Geometry: see drawing. Coordinates: mm, zero at the bounding-box minimum. Coordinates: 2 decimals unless noted, no trailing zeros. Loops run counter-clockwise (first coordinate to the right, second up) from the corner with the lowest first, then second, coordinate; pieces in that order, holes last. Notation, with made-up numbers: (-25, 11) -> (12, 11) arc R24 cw to (12, 29) -> close; hole circle Ø3 at (83.25, 8.25). An arc over 180 degrees is marked (long way). Put each result on its own line as item: value. Start each with the question number.
1) Contact query for flat-ended pins moving along their axis: P1, Ø4, axis at x = 14.5, z = 20, coming from the +Y side; P2, Ø3, axis at x = 12, z = 27, coming from the +Y side; P3, Ø3, axis at y = 4, z = 19.5, coming from the -X side. Output: stop coordinate, or through.
2) Cut plane A-A (y = 10). Return the cut outline in (x, z).
3) Material intervals for L1, parallel to Y at x = 10, z = 23.25; L2, parallel to Y at x = 17, z = 28.5; L3, parallel to X at y = 9, z = 26.5, sorted ascending.
4) Pull-direction query (X, two-part tool) for the marked faces 1 and 2; classes: pulls with the +X half, pulls with the -X half, needs draft (parallel to the pull), parting line crosses it, or undercut.
5) Cut plane C-C (z = 14.5). Return the cut outline in (x, y).
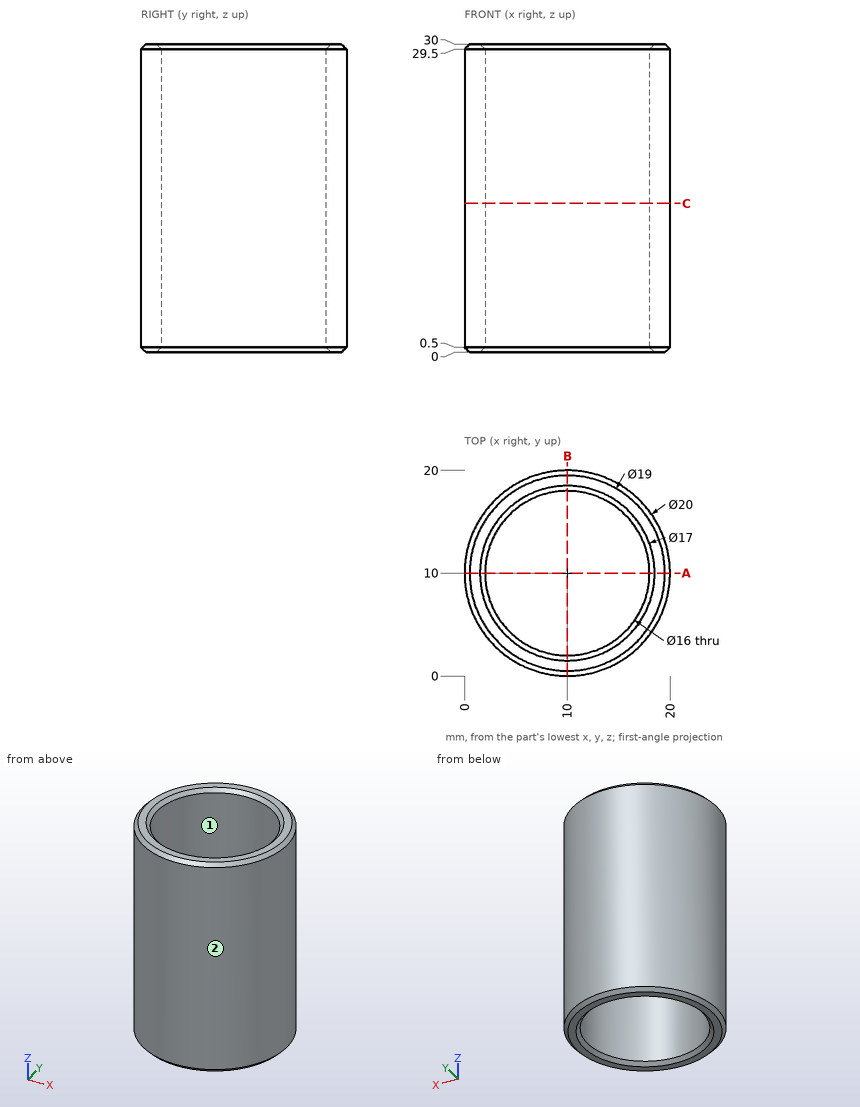
Results found:
1. P1: stops at y = 19.68
1. P2: stops at y = 19.99
1. P3: stops at x = 1.07
2. outline: (0, 0.5) -> (0.5, 0) -> (1.5, 0) -> (2, 0.5) -> (2, 29.5) -> (1.5, 30) -> (0.5, 30) -> (0, 29.5) -> close; (18, 0.5) -> (18.5, 0) -> (19.5, 0) -> (20, 0.5) -> (20, 29.5) -> (19.5, 30) -> (18.5, 30) -> (18, 29.5) -> close
3. L1: y = 0 to 2, 18 to 20
3. L2: y = 2.86 to 6.13, 13.87 to 17.14
3. L3: x = 0.05 to 2.06, 17.94 to 19.95
4. face 1: undercut
4. face 2: parting line crosses it
5. outline: circle Ø20 at (10, 10); hole circle Ø16 at (10, 10)
